```python
from build123d import *

# Parameters (mm, degrees)
F0_R     = 8
F0_W     = 1.905
F0_H     = 4.445
F0_W_2   = 4.445
F0_H_2   = 1.905
F0_W_3   = 38.1
F0_H_3   = 42.8625
F1_DEPTH = 3.175
F2_R     = 6.35
F3_R     = 5.08


with BuildPart() as f1:
    # F0 (on Top) → F1 (new body)
    with BuildSketch(Plane.XY):
        Polygon((-63.5, -31.75), (63.5, -31.75), (63.5, 31.75), (63.5, 44.45), (-63.5, 44.45), (-63.5, 31.75), align=None)
        with Locations((-44.45, -17.4625)):
            Circle(F0_R, mode=Mode.SUBTRACT)
        with Locations((-22.225, -26.19375)):
            Rectangle(F0_W, F0_H, mode=Mode.SUBTRACT)
        with Locations((-57.15, -7.9375)):
            Rectangle(F0_W_2, F0_H_2, mode=Mode.SUBTRACT)
        with Locations((-25.4, -7.9375)):
            Rectangle(F0_W_2, F0_H_2, mode=Mode.SUBTRACT)
        with Locations((22.225, -26.19375)):
            Rectangle(F0_W, F0_H, mode=Mode.SUBTRACT)
        with Locations((44.45, -17.4625)):
            Circle(F0_R, mode=Mode.SUBTRACT)
        with Locations((25.4, -7.9375)):
            Rectangle(F0_W_2, F0_H_2, mode=Mode.SUBTRACT)
        with Locations((0, 0.79375)):
            Rectangle(F0_W_3, F0_H_3, mode=Mode.SUBTRACT)
        with Locations((57.15, -7.9375)):
            Rectangle(F0_W_2, F0_H_2, mode=Mode.SUBTRACT)
        with Locations((-57.15, 26.9875)):
            Rectangle(F0_W_2, F0_H_2, mode=Mode.SUBTRACT)
        with Locations((-25.4, 26.9875)):
            Rectangle(F0_W_2, F0_H_2, mode=Mode.SUBTRACT)
        with Locations((25.4, 26.9875)):
            Rectangle(F0_W_2, F0_H_2, mode=Mode.SUBTRACT)
        with Locations((57.15, 26.9875)):
            Rectangle(F0_W_2, F0_H_2, mode=Mode.SUBTRACT)
    extrude(amount=F1_DEPTH)

    # F2
    f2_edges = [f1.edges().sort_by_distance(p)[0] for p in [
        (-19.05, 22.225, 1.5875),
        (19.05, 22.225, 1.5875),
        (-19.05, -20.6375, 1.5875),
        (19.05, -20.6375, 1.5875),
    ]]
    fillet(f2_edges, radius=F2_R)

    # F3
    f3_edges = [f1.edges().sort_by_distance(p)[0] for p in [
        (-63.5, 44.45, 1.5875),
        (-63.5, -31.75, 1.5875),
        (63.5, -31.75, 1.5875),
        (63.5, 44.45, 1.5875),
    ]]
    fillet(f3_edges, radius=F3_R)


solid = f1.part
```
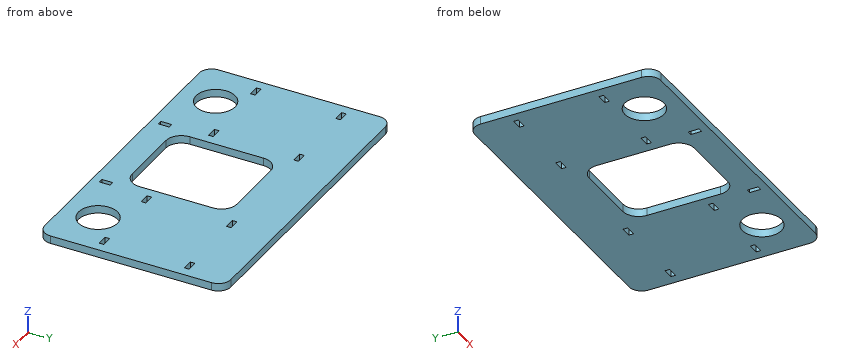
Check sheet for the modelled part. Datum: model origin and axes. Units: mm. Coordinates: 2 decimals unless noted, no trailing zeros. Loops run counter-clockwise (first coordinate to the right, second up) from the corner with the lowest first, then second, coordinate; pieces in that order, holes last.
1) Gauge pin test, flat end, axial feed: pin 1 (4 mm diameter, centred on x = -39.5, y = 9, fed in from -Z). Record the tip position at first contact, or that the pin passes through.
2) Material ranges on probe 1 along X at (y, z) = (-25.5, 1.9); probe 2 along Y at (x, z) = (-55, 1.05) (3 decimals); probe 3 along X at (y, z) = (-8, 2.35), recorded low to high.
3) Sectioned sample at C-C (z = 1.45). Count the separate pieces of the cut face and the enclosed holes in it, and give its area (3 significant figures).
4) Sectioned sample at B-B (y = 19). Record the boundary of the cut face in (x, z) (3 decimals).
Check sheet entries:
1. pin 1: stops at z = 0
2. probe 1: x = -63.5 to -23.18, -21.27 to 21.27, 23.18 to 63.5
2. probe 2: y = -31.75 to -8.89, -6.985 to 26.035, 27.94 to 44.45
2. probe 3: x = -63.5 to -59.37, -54.93 to -27.62, -23.18 to -19.05, 19.05 to 23.18, 27.62 to 54.93, 59.37 to 63.5
3. separate pieces: 1
3. enclosed holes: 13
3. area: 7,570 mm2
4. outline: (-63.5, 0) - (-18.228, 0) - (-18.228, 3.175) - (-63.5, 3.175) - close; (18.228, 0) - (63.5, 0) - (63.5, 3.175) - (18.228, 3.175) - close
